CAD build for the part. Positions are in the model's coordinates, mm. A direction names the side the tool comes from. Give positions to 0.01 mm unless a question says otherwise; leave off trailing zeros. Write each loop counter-clockwise with the first axis right and the second up, starting at its lowest first coordinate (ties: lowest second). Pieces come first, ordered by that corner, then holes. Notation, with made-up numbers: (26, -24.75) - (36, -24.75) arc R30 cw to (36, 0.25) - close; hole circle Ø6 at (55.5, 19). An arc over 180 degrees is marked (long way). Put each result on its own line as item: value. Start each with the question number.
1. Tool access for faces 1 (the cylindrical face through (5.978, 75.934, -1.374)), 2 (the flat face through (3.302, 2, -5)), 3 (the flat face through (3, -22, -73.025)): list every direction of +Z, -Z, +X, -X, +Y, -Y with a clear straight run to the whole face (end or side of a thin tool).
2. Mould opens along Z. For faces 4 (the cylindrical face through (1.628, 6.323, -1.404)), 5 (the cylindrical face through (3.256, 91.432, -1.184)), 6 (the flat face through (3, -103.855, 1)) say: +Z half, -Z half, draft (parallel to the pull), parting line (faces both ways), or undercut.
3. Cut at A-A on z = 0. List the corners of the cut face in (x, y) (3 decimals), and give its area (3 significant figures).
4. Drop flat-ended pins along their axis: pin 1 (1 mm diameter, centred on x = 6, z = -7, fed in from +Y); pin 2 (3 mm diameter, centred on x = 2, z = 10, fed in from +Y). Give the stop position or say it passes through.
5. Cut at B-B on y = 0. List the corners of the cut face in (x, z) (3 decimals), and give its area (3 significant figures).
6. Wall check: line 1 (Y direction, x = 4.3, z = 0); line 2 (Y direction, x = 5.5, z = -55); line 3 (X direction, y = 50, z = 50). Give the ranges that are in metal, low to high.
7. Cut at C-C on x = 1.5. Give the number of separate pieces and of enclosed holes in the cut face, and give its area (3 significant figures).
8. Cut at D-D on z = 55. List the corners of the cut face in (x, y), and give its area (3 significant figures).
from build123d import *

# Parameters (mm, degrees)
SKETCH1_R           = 5.08
BOSS_EXTRUDE1_DEPTH = 6.604
SKETCH2_R           = 6.477
CUT_EXTRUDE1_DEPTH  = 3.302
SKETCH3_R           = 75.946
SKETCH3_R_2         = 69.215
CUT_EXTRUDE2_DEPTH  = 1.27
SKETCH4_R           = 2.38125
CUT_EXTRUDE3_DEPTH  = 139.530727768
SKETCH6_W           = 37.512644612
SKETCH6_H           = 125.02997604
SKETCH6_W_2         = 29.936636925
CUT_EXTRUDE6_DEPTH  = 139.530727768


with BuildPart() as part:
    # Sketch1 → Boss-Extrude1 (new body)
    with BuildSketch(Plane(origin=(0, 0, 0), x_dir=(0, 0, -1), z_dir=(1, 0, 0))):
        with BuildLine():
            Line((-65.405, -103.855072673), (65.405, -103.855072673))
            ThreePointArc((65.405, -103.855072673), (70.793153673, -101.623226346), (73.025, -96.235072673))
            Line((73.025, -96.235072673), (73.025, -69.997049759))
            ThreePointArc((73.025, -69.997049759), (74.696702219, -57.072253546), (79.601785714, -44.998103417))
            ThreePointArc((79.601785714, -44.998103417), (0, 91.44), (-79.601785714, -44.998103417))
            ThreePointArc((-79.601785714, -44.998103417), (-74.696702219, -57.072253546), (-73.025, -69.997049759))
            Line((-73.025, -69.997049759), (-73.025, -96.235072673))
            ThreePointArc((-73.025, -96.235072673), (-70.793153673, -101.623226346), (-65.405, -103.855072673))
        make_face()
        with Locations(Location((0, 0, 0), (0, 0, 180))):
            Circle(SKETCH1_R, mode=Mode.SUBTRACT)
    extrude(amount=BOSS_EXTRUDE1_DEPTH)

    # Sketch2 → Cut-Extrude1 (cut)
    with BuildSketch(Plane(origin=(0, 0, 0), x_dir=(0, 0, -1), z_dir=(1, 0, 0))):
        with Locations(Location((0, 0, 0), (0, 0, 180))):
            Circle(SKETCH2_R)
    extrude(amount=CUT_EXTRUDE1_DEPTH, mode=Mode.SUBTRACT)

    # Sketch3 → Cut-Extrude2 (cut)
    with BuildSketch(Plane(origin=(6.604, 0, 0), x_dir=(0, 0, -1), z_dir=(1, 0, 0))):
        Circle(SKETCH3_R)
        Circle(SKETCH3_R_2, mode=Mode.SUBTRACT)
    extrude(amount=-CUT_EXTRUDE2_DEPTH, mode=Mode.SUBTRACT)

    # Sketch4 → Cut-Extrude3 (cut, through all)
    with BuildSketch(Plane.ZY):
        with Locations((-54.740775438, -61.789562262)):
            Circle(SKETCH4_R)
        with Locations((0, 82.55)):
            Circle(SKETCH4_R)
        with Locations((-77.185590834, -29.272633425)):
            Circle(SKETCH4_R)
        with Locations((38.362897852, 73.094394918)):
            Circle(SKETCH4_R)
        with Locations((67.93731813, 46.893744843)):
            Circle(SKETCH4_R)
        with Locations((81.948117557, 9.950302955)):
            Circle(SKETCH4_R)
        with Locations((77.185590834, -29.272633425)):
            Circle(SKETCH4_R)
        with Locations((54.740775438, -61.789562262)):
            Circle(SKETCH4_R)
        with Locations((19.755508087, -80.151247029)):
            Circle(SKETCH4_R)
        with Locations((-19.755508087, -80.151247029)):
            Circle(SKETCH4_R)
        with Locations((-81.948117557, 9.950302955)):
            Circle(SKETCH4_R)
        with Locations((-67.93731813, 46.893744843)):
            Circle(SKETCH4_R)
        with Locations((-38.362897852, 73.094394918)):
            Circle(SKETCH4_R)
    extrude(amount=-CUT_EXTRUDE3_DEPTH, mode=Mode.SUBTRACT)

    # Sketch6 → Cut-Extrude6 (cut, through all)
    with BuildSketch(Plane(origin=(6.604, 0, 0), x_dir=(0, 0, -1), z_dir=(1, 0, 0))):
        with Locations((-91.781322306, -7.482061739)):
            Rectangle(SKETCH6_W, SKETCH6_H)
        with Locations((87.993318463, -7.482061739)):
            Rectangle(SKETCH6_W_2, SKETCH6_H)
    extrude(amount=-CUT_EXTRUDE6_DEPTH, mode=Mode.SUBTRACT)


solid = part.part
Report:
1. face 1: +X
1. face 2: -X
1. face 3: -Z, +X, -X, +Y, -Y
2. face 4: undercut
2. face 5: parting line
2. face 6: draft
3. outline: (0, -103.855) - (6.604, -103.855) - (6.604, -75.946) - (5.334, -75.946) - (5.334, -69.215) - (6.604, -69.215) - (6.604, -5.08) - (3.302, -5.08) - (3.302, -6.477) - (0, -6.477) - close; (0, 6.477) - (3.302, 6.477) - (3.302, 5.08) - (6.604, 5.08) - (6.604, 69.215) - (5.334, 69.215) - (5.334, 75.946) - (6.604, 75.946) - (6.604, 80.169) - (0, 80.169) - close; (0, 84.931) - (6.604, 84.931) - (6.604, 91.44) - (0, 91.44) - close
3. area: 1,160 mm²
4. pin 1: stops at y = 91.21
4. pin 2: stops at y = 91.04
5. outline: (0, -73.025) - (5.334, -73.025) - (5.334, -69.215) - (6.604, -69.215) - (6.604, -5.08) - (3.302, -5.08) - (3.302, -6.477) - (0, -6.477) - close; (0, 6.477) - (3.302, 6.477) - (3.302, 5.08) - (6.604, 5.08) - (6.604, 69.215) - (5.334, 69.215) - (5.334, 73.025) - (0, 73.025) - close
5. area: 879 mm²
6. line 1: y = -103.86 to -5.08, 5.08 to 80.17, 84.93 to 91.44
6. line 2: y = -103.86 to -64.16, -59.42 to -52.37, -42.02 to 42.02, 52.37 to 73.05
6. line 3: x = 0 to 5.33
7. separate pieces: 1
7. enclosed holes: 10
7. area: 26,600 mm²
8. outline: (0, -103.86) - (6.6, -103.86) - (6.6, -64.16) - (0, -64.16) - close; (0, -59.42) - (6.6, -59.42) - (6.6, -52.37) - (5.33, -52.37) - (5.33, -42.02) - (6.6, -42.02) - (6.6, 42.02) - (5.33, 42.02) - (5.33, 52.37) - (6.6, 52.37) - (6.6, 73.05) - (0, 73.05) - close
8. area: 1,110 mm²
